Part model, mm, in its own coordinate system. A direction names the side the tool comes from. Round coordinates to 2 decimals unless told otherwise and drop trailing zeros. Write each loop counter-clockwise with the first axis right and the second up, starting at its lowest first coordinate (ties: lowest second). Pieces come first, ordered by that corner, then holes. Notation, with made-up numbers: M -33.5,8.25 L 4.5,8.25 A29 ccw 4.5,46.25 Z; hole C -13.75,20.25 d7. An arc over 180 degrees is marked long. Use a Markdown table: item, result. Add a question column.
1) Drop flat-ended pins along their axis: P1, Ø2.5, axis at x = -16.5, y = 1.5, coming from the -Z side; P2, Ø2.5, axis at x = 32.5, y = 2.5, coming from the -Z side; P3, Ø1.5, axis at y = 2, z = 100.5, coming from the -X side. Give the stop position or say it passes through.
2) Slice it at B-B on y = 1.95. Give the number of separate pieces and of enclosed holes in the cut face, plus the area to 3 significant figures.
3) Two-plate mould, pull along Z, no slides. Class faces 1 (the face through (-9.392, 2.504, -112.855)), 2 (the face through (44, 0, 104)), 3 (the face through (15.18, 2.58, 126.28)): released by +Z, released by -Z, zero draft, split by the parting line, or undercut.
4) Slice it at A-A on z = -6. Write the cut outline in (x, y).
5) Which spindle directions (+Z, -Z, +X, -X, +Y, -Y) get a long thin tool onto all of the face, cutting with end or side? Do faces 4 (the face through (44, 5.08, 104)), 5 (the face through (15.38, 2.58, 196.9)). Say none if no direction does.
6) Wall check: probe 1 along Z at (x, y) = (56, 0.7); probe 2 along Z at (x, y) = (30.5, 0.55); probe 3 along X at (y, z) = (2.1, 13). Give the ranges that are in metal, low to high.
```python
from build123d import *

# Parameters (mm, degrees)
BOSS_EXTRUDE1_DEPTH = 5.08
SKETCH3_W           = 20.066
SKETCH3_H           = 39.624
CUT_EXTRUDE1_DEPTH  = 5.08
SKETCH4_R           = 2.159
CUT_EXTRUDE2_DEPTH  = 5.08
CUT_EXTRUDE3_DEPTH  = 5.08
SKETCH6_W           = 5.08
SKETCH6_H           = 25.4
CUT_EXTRUDE4_DEPTH  = 5.08
SKETCH7_W           = 5.08
SKETCH7_H           = 25.4
CUT_EXTRUDE5_DEPTH  = 5.08
SKETCH8_W           = 5.08
SKETCH8_H           = 25.4
CUT_EXTRUDE6_DEPTH  = 5.08
SKETCH9_W           = 5.08
SKETCH9_H           = 25.4
CUT_EXTRUDE7_DEPTH  = 5.08
SKETCH10_W          = 25.4
SKETCH10_H          = 5.08
CUT_EXTRUDE8_DEPTH  = 5.08
SKETCH11_W          = 25.4
SKETCH11_H          = 5.08
CUT_EXTRUDE9_DEPTH  = 5.08
SKETCH12_R          = 1.27
CUT_EXTRUDE10_DEPTH = 5.08
SKETCH13_W          = 10.16
SKETCH13_H          = 5.08
CUT_EXTRUDE11_DEPTH = 5.08
SKETCH14_W          = 7.62
SKETCH14_H          = 7.62
CUT_EXTRUDE12_DEPTH = 5.08
SKETCH15_R          = 1.905
CUT_EXTRUDE13_DEPTH = 5.08
SKETCH16_R          = 2.49555
CUT_EXTRUDE14_DEPTH = 5.08


with BuildPart() as part:
    # Sketch2 → Boss-Extrude1 (new body)
    with BuildSketch(Plane(origin=(0, 0, 0), x_dir=(1, 0, 0), z_dir=(0, 1, 0))):
        Polygon((-19.05, -71.23934806), (-19.05, -249.03934806), (107.95, -249.03934806), (107.95, -60.96), (107.95, 0), (0, 0), (0, 65.786), (0, 97.473109619), (0, 116.165799875), (-19.05, 109.450065503), align=None)
    extrude(amount=BOSS_EXTRUDE1_DEPTH)

    # Sketch3 → Cut-Extrude1 (cut)
    with BuildSketch(Plane(origin=(0, 5.08, 0), x_dir=(1, 0, 0), z_dir=(0, 1, 0))):
        with Locations((90.297, -37.703734372)):
            Rectangle(SKETCH3_W, SKETCH3_H)
    extrude(amount=-CUT_EXTRUDE1_DEPTH, mode=Mode.SUBTRACT)

    # Sketch4 → Cut-Extrude2 (cut)
    with BuildSketch(Plane(origin=(0, 5.08, 0), x_dir=(1, 0, 0), z_dir=(0, 1, 0))):
        with Locations((83.82, -13.573734372)):
            Circle(SKETCH4_R)
        with Locations((96.52, -13.573734372)):
            Circle(SKETCH4_R)
        with Locations((83.82, -61.833734372)):
            Circle(SKETCH4_R)
        with Locations((96.52, -61.833734372)):
            Circle(SKETCH4_R)
    extrude(amount=-CUT_EXTRUDE2_DEPTH, mode=Mode.SUBTRACT)

    # Sketch5 → Cut-Extrude3 (cut)
    with BuildSketch(Plane(origin=(0, 5.08, 0), x_dir=(1, 0, 0), z_dir=(0, 1, 0))):
        with BuildLine():
            Line((24.257, -122.461402467), (64.611105155, -122.461402467))
            ThreePointArc((64.611105155, -122.461402467), (73.591361276, -126.181146346), (77.311105155, -135.161402467))
            Line((77.311105155, -135.161402467), (77.311105155, -187.819065756))
            ThreePointArc((77.311105155, -187.819065756), (73.591361276, -196.799321877), (64.611105155, -200.519065756))
            Line((64.611105155, -200.519065756), (24.257, -200.519065756))
            ThreePointArc((24.257, -200.519065756), (15.276743879, -196.799321877), (11.557, -187.819065756))
            Line((11.557, -187.819065756), (11.557, -135.161402467))
            ThreePointArc((11.557, -135.161402467), (15.276743879, -126.181146346), (24.257, -122.461402467))
        make_face()
    extrude(amount=-CUT_EXTRUDE3_DEPTH, mode=Mode.SUBTRACT)

    # Sketch6 → Cut-Extrude4 (cut)
    with BuildSketch(Plane(origin=(0, 5.08, 0), x_dir=(1, 0, 0), z_dir=(0, 1, 0))):
        with Locations((105.41, -224.90934806)):
            Rectangle(SKETCH6_W, SKETCH6_H)
    extrude(amount=-CUT_EXTRUDE4_DEPTH, mode=Mode.SUBTRACT)

    # Sketch7 → Cut-Extrude5 (cut)
    with BuildSketch(Plane(origin=(0, 5.08, 0), x_dir=(1, 0, 0), z_dir=(0, 1, 0))):
        with Locations((105.41, -181.72934806)):
            Rectangle(SKETCH7_W, SKETCH7_H)
    extrude(amount=-CUT_EXTRUDE5_DEPTH, mode=Mode.SUBTRACT)

    # Sketch8 → Cut-Extrude6 (cut)
    with BuildSketch(Plane(origin=(0, 5.08, 0), x_dir=(1, 0, 0), z_dir=(0, 1, 0))):
        with Locations((105.41, -138.54934806)):
            Rectangle(SKETCH8_W, SKETCH8_H)
        with Locations((105.41, -95.36934806)):
            Rectangle(SKETCH8_W, SKETCH8_H)
    extrude(amount=-CUT_EXTRUDE6_DEPTH, mode=Mode.SUBTRACT)

    # Sketch9 → Cut-Extrude7 (cut)
    with BuildSketch(Plane(origin=(0, 5.08, 0), x_dir=(1, 0, 0), z_dir=(0, 1, 0))):
        with Locations((-16.51, -224.90934806)):
            Rectangle(SKETCH9_W, SKETCH9_H)
        with Locations((-16.51, -181.72934806)):
            Rectangle(SKETCH9_W, SKETCH9_H)
        with Locations((-16.51, -138.54934806)):
            Rectangle(SKETCH9_W, SKETCH9_H)
        with Locations((-16.51, -95.36934806)):
            Rectangle(SKETCH9_W, SKETCH9_H)
    extrude(amount=-CUT_EXTRUDE7_DEPTH, mode=Mode.SUBTRACT)

    # Sketch10 → Cut-Extrude8 (cut)
    with BuildSketch(Plane(origin=(0, 5.08, 0), x_dir=(1, 0, 0), z_dir=(0, 1, 0))):
        with Locations((6.35, -73.77934806)):
            Rectangle(SKETCH10_W, SKETCH10_H)
        with Locations((44.45, -73.77934806)):
            Rectangle(SKETCH10_W, SKETCH10_H)
        with Locations((82.55, -73.77934806)):
            Rectangle(SKETCH10_W, SKETCH10_H)
    extrude(amount=-CUT_EXTRUDE8_DEPTH, mode=Mode.SUBTRACT)

    # Sketch11 → Cut-Extrude9 (cut)
    with BuildSketch(Plane(origin=(0, 5.08, 0), x_dir=(1, 0, 0), z_dir=(0, 1, 0))):
        with Locations((6.35, -246.49934806)):
            Rectangle(SKETCH11_W, SKETCH11_H)
        with Locations((44.45, -246.49934806)):
            Rectangle(SKETCH11_W, SKETCH11_H)
        with Locations((82.55, -246.49934806)):
            Rectangle(SKETCH11_W, SKETCH11_H)
    extrude(amount=-CUT_EXTRUDE9_DEPTH, mode=Mode.SUBTRACT)

    # Sketch12 → Cut-Extrude10 (cut)
    with BuildSketch(Plane(origin=(0, 5.08, 0), x_dir=(1, 0, 0), z_dir=(0, 1, 0))):
        with Locations((-14.998025324, 105.700929136)):
            Circle(SKETCH12_R)
        with Locations((-4.064, 105.700929136)):
            Circle(SKETCH12_R)
    extrude(amount=-CUT_EXTRUDE10_DEPTH, mode=Mode.SUBTRACT)

    # Sketch13 → Cut-Extrude11 (cut)
    with BuildSketch(Plane(origin=(0, 5.08, 0), x_dir=(1, 0, 0), z_dir=(0, 1, 0))):
        with Locations((20.32, -45.974710139)):
            Rectangle(SKETCH13_W, SKETCH13_H)
        with Locations((40.64, -45.974710139)):
            Rectangle(SKETCH13_W, SKETCH13_H)
    extrude(amount=-CUT_EXTRUDE11_DEPTH, mode=Mode.SUBTRACT)

    # Sketch14 → Cut-Extrude12 (cut)
    with BuildSketch(Plane(origin=(0, 5.08, 0), x_dir=(1, 0, 0), z_dir=(0, 1, 0))):
        with Locations((31.877, -58.119790423)):
            Rectangle(SKETCH14_W, SKETCH14_H)
    extrude(amount=-CUT_EXTRUDE12_DEPTH, mode=Mode.SUBTRACT)

    # Sketch15 → Cut-Extrude13 (cut)
    with BuildSketch(Plane(origin=(0, 5.08, 0), x_dir=(1, 0, 0), z_dir=(0, 1, 0))):
        with Locations((-9.5377, 71.350065503)):
            Circle(SKETCH15_R)
        with Locations((-9.5377, -4.849934497)):
            Circle(SKETCH15_R)
    extrude(amount=-CUT_EXTRUDE13_DEPTH, mode=Mode.SUBTRACT)

    # Sketch16 → Cut-Extrude14 (cut)
    with BuildSketch(Plane(origin=(0, 5.08, 0), x_dir=(1, 0, 0), z_dir=(0, 1, 0))):
        with Locations((38.354, -109.869872905)):
            Circle(SKETCH16_R)
        with Locations((50.658638695, -109.869872905)):
            Circle(SKETCH16_R)
    extrude(amount=-CUT_EXTRUDE14_DEPTH, mode=Mode.SUBTRACT)


solid = part.part
```
Entries:
| question | item | result |
|---|---|---|
| 1 | P1 | stops at z = -110.79 |
| 1 | P2 | stops at z = 0 |
| 1 | P3 | stops at x = -13.97 |
| 2 | separate pieces | 1 |
| 2 | enclosed holes | 18 |
| 2 | area | 25,900 mm^2 |
| 3 | face 1 | released by -Z |
| 3 | face 2 | zero draft |
| 3 | face 3 | undercut |
| 4 | outline | M -19.05,0 L 0,0 L 0,5.08 L -19.05,5.08 Z |
| 5 | face 4 | +Z, -Z, +X, -X, +Y |
| 5 | face 5 | +Y, -Y |
| 6 | probe 1 | z = 0 to 71.24, 76.32 to 122.46, 200.52 to 243.96 |
| 6 | probe 2 | z = 0 to 54.31, 61.93 to 122.46, 200.52 to 249.04 |
| 6 | probe 3 | x = -19.05 to 81.74, 85.9 to 94.44, 98.6 to 107.95 |
